Can you work these out from the drawing? Everything is in mm from the part's minimum corner. Coordinates: 2 decimals unless noted, no trailing zeros. Order: outer loops, then holes, each group sorted by start corner. A loop starts at its lowest first (then second) coordinate and runs counter-clockwise, first axis right, second up. Notation, with made-up numbers: (31.5, 56) - (36.5, 56) arc R21 ccw to (36.5, 90) - close; hole circle Ø11 at (-6, -24). An arc over 180 degrees is marked (long way). One line per item, written item: value.
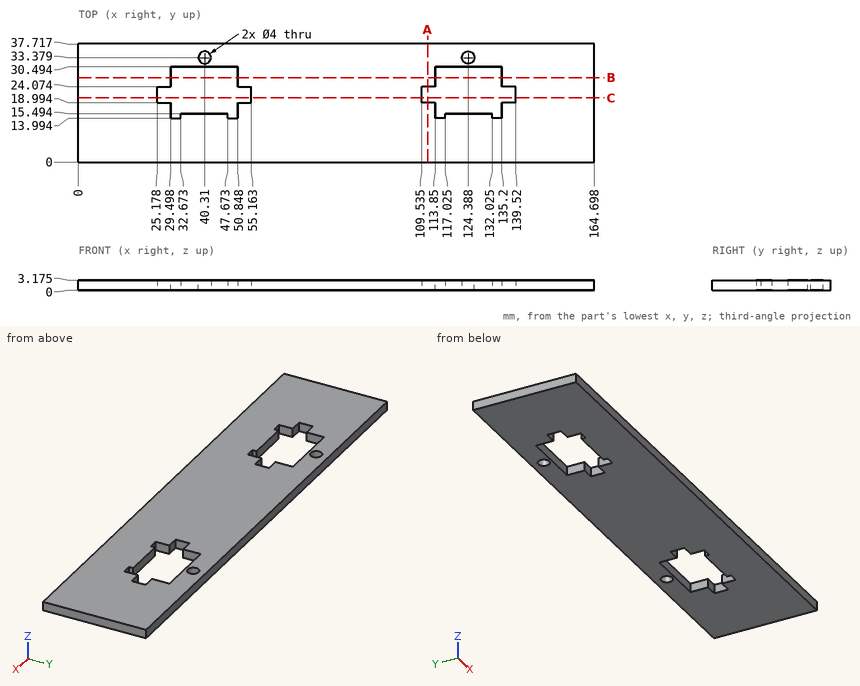
Item 1: I want a section at C-C on y = 20.5. Please give me the cut outline in (x, z) (1 decimal).
Conclusion:
outline: (0, 0) - (25.2, 0) - (25.2, 3.2) - (0, 3.2) - close; (55.2, 0) - (109.5, 0) - (109.5, 3.2) - (55.2, 3.2) - close; (139.5, 0) - (164.7, 0) - (164.7, 3.2) - (139.5, 3.2) - close
Item 2: If I drill on probe 1 along X at (y, z) = (29, 1.85); probe 2 along Y at (x, z) = (138, 1.45); probe 3 along Y at (x, z) = (48, 2.75), over which ranges is the centre line in solid material (lowest first)?
Conclusion:
probe 1: 0 to 29.5, 50.85 to 113.85, 135.2 to 164.7
probe 2: 0 to 18.99, 24.07 to 37.72
probe 3: 0 to 13.99, 30.49 to 37.72
Item 3: I'm going to push a flat-ended pin straight in: pin 1 Ø1 at (x, z) = (138, 1) entering from -Y. Where does the tip first touch, or does it pass through?
Conclusion:
pin 1: y = 0
Item 4: I want a section at A-A on x = 111.5. Please give me the cut outline in (y, z) (1 decimal).
Conclusion:
outline: (0, 0) - (19, 0) - (19, 3.2) - (0, 3.2) - close; (24.1, 0) - (37.7, 0) - (37.7, 3.2) - (24.1, 3.2) - close
Item 5: I want a section at B-B on y = 27. Give the number of separate pieces and of enclosed holes in the cut face.
Conclusion:
separate pieces: 3
enclosed holes: 0
